```python
from build123d import *

# Parameters (mm, degrees)
SALIENTE_EXTRUIR1_DEPTH = 200
CROQUIS2_R              = 6
CORTAR_EXTRUIR1_DEPTH   = 400


with BuildPart() as part:
    # Croquis1 → Saliente-Extruir1 (new, symmetric)
    with BuildSketch(Plane.XY):
        Polygon((-10.469747898, -27.240151607), (-10.469747898, -35.650909673), (-14.818838224, -40), (-24.971054909, -40), (-30, -34.971054909), (-30, 32.215207139), (-24.971054909, 40), (25.20346735, 40), (30, 32.215207139), (30, -35.650909673), (25.650909673, -40), (14.472500162, -40), (10.123409835, -35.650909673), (10.123409835, -27.240151607), (13.123409835, -27.240151607), (13.123409835, -34.408268986), (15.715140849, -37), (24.408268986, -37), (27, -34.408268986), (27, 31.365191547), (23.528161609, 37), (-23.337516983, 37), (-27, 31.330486588), (-27, -33.728414222), (-23.728414222, -37), (-16.061478911, -37), (-13.469747898, -34.408268986), (-13.469747898, -27.240151607), align=None)
    extrude(amount=SALIENTE_EXTRUIR1_DEPTH, both=True)

    # Croquis2 → Cortar-Extruir1 (cut)
    with BuildSketch(Plane(origin=(0, 40, 0), x_dir=(1, 0, 0), z_dir=(0, 1, 0))):
        with Locations(Location((0, 170, 0), (0, 0, 270))):
            Circle(CROQUIS2_R)
        with Locations(Location((0, -170, 0), (0, 0, 270))):
            Circle(CROQUIS2_R)
    extrude(amount=-CORTAR_EXTRUIR1_DEPTH, mode=Mode.SUBTRACT)


solid = part.part
```
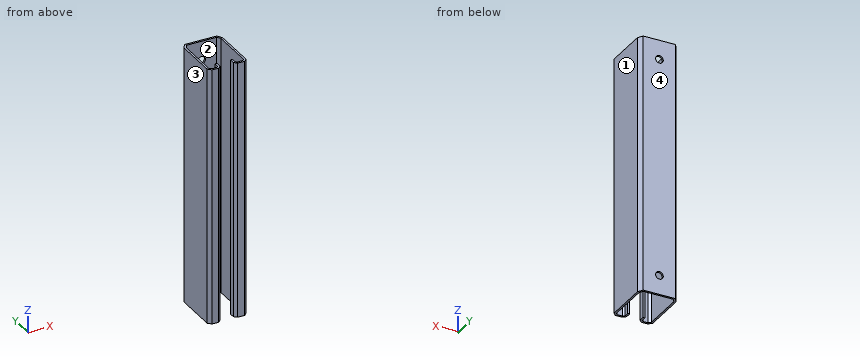
Geometry check sheet. Reference: the model listing, model coordinates, mm. Face numbers are marked on the shaded views. Give positions to 0.01 mm unless a question says otherwise; leave off trailing zeros. Write each loop counter-clockwise with the first axis right and the second up, starting at its lowest first coordinate (ties: lowest second). Pieces come first, ordered by that corner, then holes.
1) Section check B-B, the plane y = -21. Record the boundary of the cut face in (x, z), and give its area (3 significant figures).
2) Release check for a two-part mould opening along X. For the marked faces 1, 2, 3 and 4 record: pulls with the +X half, pulls with the -X half, needs draft (parallel to the pull), parting line crosses it, or undercut.
3) Section check A-A, the plane x = 19.5. Record the boundary of the cut face in (y, z), and give its area (3 significant figures).
4) Material ranges on L1, parallel to X at y = -20, z = -143; L2, parallel to X at y = -31.5, z = 51.5; L3, parallel to Y at x = -19, z = 8.5, recorded low to high.
5) Gauge pin test, flat ends, axial feed: pin 1 (23.5 mm diameter, centred on x = 10.5, z = -74.5, fed in from -Y); pin 2 (15.5 mm diameter, centred on x = 0, z = -170, fed in from -Y). Record the tip position at first contact, or that the pin passes through.
6) Section check D-D, the plane x = 0. Record the boundary of the cut face in (y, z), and give its area (3 significant figures).
Computed:
1. outline: (-30, -200) - (-27, -200) - (-27, 200) - (-30, 200) - close; (27, -200) - (30, -200) - (30, 200) - (27, 200) - close
1. area: 2,400 mm2
2. face 1: pulls with the +X half
2. face 2: undercut
2. face 3: pulls with the -X half
2. face 4: needs draft
3. outline: (-40, -200) - (-37, -200) - (-37, 200) - (-40, 200) - close; (37, -200) - (40, -200) - (40, 200) - (37, 200) - close
3. area: 2,400 mm2
4. L1: x = -30 to -27, 27 to 30
4. L2: x = -30 to -27, -13.47 to -10.47, 10.12 to 13.12, 27 to 30
4. L3: y = -40 to -37, 37 to 40
5. pin 1: stops at y = -40
5. pin 2: stops at y = 37
6. outline: (37, -200) - (40, -200) - (40, -176) - (37, -176) - close; (37, -164) - (40, -164) - (40, 164) - (37, 164) - close; (37, 176) - (40, 176) - (40, 200) - (37, 200) - close
6. area: 1,130 mm2
